Work out the finished part from the listing and answer in its coordinate system (mm). A direction names the side the tool comes from. Give positions to 0.01 mm unless a question says otherwise; leave off trailing zeros. Loops run counter-clockwise (first coordinate to the right, second up) from the corner with the lowest first, then second, coordinate; pieces in that order, holes last. Notation, with made-up numbers: M 37,37 L 94,37 A17 cw 94,55 Z; hole C 86.25,30.25 d11. An arc over 180 degrees is marked long. Use a Markdown table: item, result.
```python
from build123d import *

# Parameters (mm, degrees)
AUFSATZ_LINEAR_AUSTRAGEN2_DEPTH             = 17.5
SKIZZE3_R                                   = 1.5
SKIZZE3_W                                   = 41.5
SKIZZE3_H                                   = 20
SCHNITT_LINEAR_AUSTRAGEN1_DEPTH             = 4
SKIZZE4_W                                   = 74
SKIZZE4_H                                   = 3
AUFSATZ_LINEAR_AUSTRAGEN3_DEPTH             = 3
AUFSATZ_LINEAR_AUSTRAGEN4_DEPTH             = 3
FORMSENKUNG_F_R_M3_SENKSCHRAUBE_MIT_2_COUNT = 2
FORMSENKUNG_F_R_M3_SENKSCHRAUBE_MIT_2_PITCH = 12
SKIZZE8_R                                   = 2.25
SCHNITT_LINEAR_AUSTRAGEN2_DEPTH             = 74


with BuildPart() as part:
    # Skizze2 → Aufsatz-Linear austragen2 (new body, symmetric)
    with BuildSketch(Plane(origin=(0, 0, 0), x_dir=(1, 0, 0), z_dir=(0, 1, 0))):
        Polygon((-40, 0), (40, 0), (40, -6), (37, -6), (37, -3), (-37, -3), (-37, -6), (-40, -6), align=None)
    extrude(amount=AUFSATZ_LINEAR_AUSTRAGEN2_DEPTH, both=True)

    # Skizze3 → Schnitt-Linear austragen1 (cut, through all)
    with BuildSketch(Plane.XY.offset(3)):
        with Locations((-34.25, -2.5)):
            Circle(SKIZZE3_R)
        with Locations((-34.25, -12.5)):
            Circle(SKIZZE3_R)
        with Locations((14.25, -2.5)):
            Circle(SKIZZE3_R)
        with Locations((14.25, -12.5)):
            Circle(SKIZZE3_R)
        with Locations((-10, -7.5)):
            Rectangle(SKIZZE3_W, SKIZZE3_H)
    extrude(amount=-SCHNITT_LINEAR_AUSTRAGEN1_DEPTH, mode=Mode.SUBTRACT)

    # Skizze4 → Aufsatz-Linear austragen3 (add)
    with BuildSketch(Plane.XY.offset(3)):
        with Locations((0, 16)):
            Rectangle(SKIZZE4_W, SKIZZE4_H)
    extrude(amount=AUFSATZ_LINEAR_AUSTRAGEN3_DEPTH)

    # Skizze5 → Aufsatz-Linear austragen4 (add)
    with BuildSketch(Plane.XZ.offset(17.5)):
        Polygon((-37, 6), (-34.992640687, 6), (-29.992640687, 11), (9.992640687, 11), (14.992640687, 6), (37, 6), (37, 3), (10.75, 3), (10.75, 6), (8.75, 8), (-28.75, 8), (-30.75, 6), (-30.75, 3), (-37, 3), align=None)
    extrude(amount=-AUFSATZ_LINEAR_AUSTRAGEN4_DEPTH)

    # Skizze6 → Formsenkung für M3 Senkschraube mit Innensechskant1 (revolve, cut)
    with BuildSketch(Plane(origin=(-37, 6, 3.5), x_dir=(0, 0, -1), z_dir=(0, 1, 0))):
        Polygon((0, 0), (0, 3), (0.8, 3), (0.8, 0.95), (1.75, 0), align=None)
    formsenkung_f_r_m3_senkschraube_mit_inne = revolve(axis=Axis((-30.65, 6, 3.5), (-1, 0, 0)), mode=Mode.SUBTRACT)

    # Formsenkung f_r M3 Senkschraube mit  2: Formsenkung für M3 Senkschraube mit Innensechskant1 ×2
    with Locations(*[(0, -i * FORMSENKUNG_F_R_M3_SENKSCHRAUBE_MIT_2_PITCH, 0) for i in range(1, FORMSENKUNG_F_R_M3_SENKSCHRAUBE_MIT_2_COUNT)]):
        add(formsenkung_f_r_m3_senkschraube_mit_inne, mode=Mode.SUBTRACT)

    # Skizze8 → Schnitt-Linear austragen2 (cut)
    with BuildSketch(Plane(origin=(-37, 0, 0), x_dir=(0, 0, -1), z_dir=(1, 0, 0))):
        with Locations((-3.5, -6)):
            Circle(SKIZZE8_R)
        with Locations((-3.5, 6)):
            Circle(SKIZZE8_R)
    extrude(amount=SCHNITT_LINEAR_AUSTRAGEN2_DEPTH, mode=Mode.SUBTRACT)

    # Spiegeln2: Formsenkung für M3 Senkschraube mit Innensechskant1 across plane
    add(formsenkung_f_r_m3_senkschraube_mit_inne.mirror(Plane(origin=(0, 0, 0), x_dir=(0, 0, 1), z_dir=(1, 0, 0))), mode=Mode.SUBTRACT)

    # Spiegeln2 copy 1 sketch → Spiegeln2 copy 1 (revolve, cut)
    with BuildSketch(Plane(origin=(37, -6, 3.5), x_dir=(0, 0, -1), z_dir=(0, 1, 0))):
        Polygon((0, 0), (0, -3), (0.8, -3), (0.8, -0.95), (1.75, 0), align=None)
    revolve(axis=Axis((30.65, -6, 3.5), (-1, 0, 0)), mode=Mode.SUBTRACT)


solid = part.part
```
(1) A cutting plane is placed at D-D (x = 23). Write down the section's boundary in (y, z).
Entries:
| item | result |
|---|---|
| outline | M -17.5,0 L 17.5,0 L 17.5,6 L 14.5,6 L 14.5,3 L 8.19,3 A2.25 cw 3.81,3 L -3.81,3 A2.25 cw -8.19,3 L -14.5,3 L -14.5,6 L -17.5,6 Z |
(2) Given P1, Ø6, axis at x = 15.5, y = 1, coming from the +Z side; P2, Ø3.5, axis at x = -34.25, y = -12.5, coming from the -Z side; P3, Ø2.5, axis at x = -34.25, y = -2.5, coming from the +Z side; P4, Ø6, axis at x = 5, y = -13, coming from the -Z side, each flat-ended and moving along its own axis, determine where each tip first touches the part or whether it passes through.
Entries:
| item | result |
|---|---|
| P1 | stops at z = 3 |
| P2 | stops at z = 0 |
| P3 | passes through |
| P4 | stops at z = 8 |
(3) A cutting plane is placed at B-B (x = -26.5). Write down the section's boundary in (y, z), and give its area (3 significant figures).
Entries:
| item | result |
|---|---|
| outline | M -17.5,8 L -14.5,8 L -14.5,11 L -17.5,11 Z; M 2.5,0 L 17.5,0 L 17.5,6 L 14.5,6 L 14.5,3 L 8.19,3 A2.25 cw 3.81,3 L 2.5,3 Z |
| area | 57.3 mm² |
(4) A cutting plane is placed at A-A (y = -6). Write down the section's boundary in (x, z), and give its area (3 significant figures).
Entries:
| item | result |
|---|---|
| outline | M -40,0 L -30.75,0 L -30.75,1.25 L -37,1.25 L -37,1.75 L -37.95,2.7 L -40,2.7 Z; M -40,4.3 L -37.95,4.3 L -37,5.25 L -37,6 L -40,6 Z; M 10.75,0 L 40,0 L 40,2.7 L 37.95,2.7 L 37,1.75 L 37,1.25 L 10.75,1.25 Z; M 37,5.25 L 37.95,4.3 L 40,4.3 L 40,6 L 37,6 Z |
| area | 65.2 mm² |
(5) Consider probe 1 along X at (y, z) = (-2.5, 2); probe 2 along Y at (x, z) = (39.5, 3.5); probe 3 along Y at (x, z) = (-35.5, 5). Determine where each line is inside the solid, lowest interval first. Write a range as [from, to].
Entries:
| item | result |
|---|---|
| probe 1 | x = [-40, -35.75], [-32.75, -30.75], [10.75, 12.75], [15.75, 40] |
| probe 2 | y = [-17.5, -6.8], [-5.2, 5.2], [6.8, 17.5] |
| probe 3 | y = [-17.5, -14.5], [14.5, 17.5] |
(6) A cutting plane is placed at C-C (y = 13.5). Write down the section's boundary in (x, z), and give its area (3 significant figures).
Entries:
| item | result |
|---|---|
| outline | M -40,0 L 40,0 L 40,6 L 37,6 L 37,3 L -37,3 L -37,6 L -40,6 Z |
| area | 258 mm² |
(7) The mould has two halves that part along Z. Classify faces 3 (the flat face through (1, -17.5, 9)), 4 (the cylindrical face through (38.96, 6.49, 4.13)), 5 (the flat face through (-10, -16, 8)): released by +Z, released by -Z, zero draft, split by the parting line, or undercut.
Entries:
| item | result |
|---|---|
| face 3 | zero draft |
| face 4 | undercut |
| face 5 | released by -Z |
(8) Which of the six approach directions +Z, -Z, +X, -X, +Y, -Y give full straight-line access (tool end or side, diameter ignored) to faces 1 (the cylindrical face through (14.055, -1.013, 1.521)), 2 (the flat face through (-33.8, -10.6, 3))?
Entries:
| item | result |
|---|---|
| face 1 | +Z, -Z |
| face 2 | +Z |
